For this review, take the finished solid that the model builds, in its own axes (mm). A direction names the side the tool comes from. Round coordinates to 2 decimals unless told otherwise and drop trailing zeros. Loops run counter-clockwise (first coordinate to the right, second up) from the corner with the lowest first, then second, coordinate; pieces in that order, holes last.
1) Mouldability with a two-part tool opening along X and no side actions: class faces 1 (the cylindrical face through (-26, 84, 46)), 2 (the cylindrical face through (4.99, 81.15, 45.94)), 3 (the flat face through (0, 44, 50)) as pulls with the +X half, pulls with the -X half, needs draft (parallel to the pull), parting line crosses it, or undercut.
2) Take a section at B-B (x = -3). State the section outline as (y, z) points.
3) Wall thickness on L1, parallel to Y at x = 5.5, z = 19.5; L2, parallel to Z at x = -15.5, y = 79.5; L3, parallel to X at y = 14.5, z = 48: over which ranges is each line inside the solid? List them lowest first.
4) Take a section at D-D (y = 24.5). State the section outline as (x, z) points.
5) Take a section at C-C (z = 15). State the section outline as (x, y) points, then the cut area to 3 significant figures.
6) Insertion check: pin 1 (5 mm diameter, centred on x = -10, y = 15, fed in from +Z); pin 2 (9 mm diameter, centred on x = -24.5, y = 73.5, fed in from +Z); pin 3 (2.5 mm diameter, centred on x = 0.5, y = -2.5, fed in from -Z); pin 4 (5.5 mm diameter, centred on y = -2, z = 14, fed in from -X). Each pin has a flat end and moves straight along its axis. Give the tip position at first contact, or say it passes through.
7) Take a section at A-A (y = 72.5). State the section outline as (x, z) points, then the cut area to 3 significant figures.
8) Tool access review of faces 4 (the flat face through (-48, 72, 46)), 5 (the flat face through (-37, 72, 49.025)), 6 (the cylindrical face through (-26, 60, 46)), 7 (the flat face through (-37, 72, 43.025)): name each direction out of +Z, -Z, +X, -X, +Y, -Y from which nothing blocks a thin tool from reaching the whole face with its end or side.
```python
from build123d import *

# Parameters (mm, degrees)
ARM_FEATURE_SKETCH_W = 16
ARM_FEATURE_SKETCH_H = 8
ARM_FEATURE_DEPTH    = 50
TAB_FEATURE_SKETCH_W = 8
TAB_FEATURE_SKETCH_H = 25
TAB_FEATURE_DEPTH    = 5
LEG_FEATURE_SKETCH_W = 16
LEG_FEATURE_SKETCH_H = 8
LEG_FEATURE_DEPTH    = 80
SLOT_FEATURE_DEPTH   = 42
STRAP_FEATURE_DEPTH  = 6
STRAP_CUT_SKETCH_W   = 4
STRAP_CUT_SKETCH_H   = 20
STRAP_CUT_DEPTH      = 6
FILLET1_R            = 10
FILLET2_R            = 10
FILLET3_R            = 10


with BuildPart() as part:
    # Arm Feature Sketch → Arm Feature (new body)
    with BuildSketch(Plane.XY):
        Rectangle(ARM_FEATURE_SKETCH_W, ARM_FEATURE_SKETCH_H)
    extrude(amount=ARM_FEATURE_DEPTH)

    # Tab Feature Sketch → Tab Feature (cut)
    with BuildSketch(Plane(origin=(0, -4, 0), x_dir=(1, 0, 0), z_dir=(0, 1, 0))):
        with Locations((0, -12.5)):
            Rectangle(TAB_FEATURE_SKETCH_W, TAB_FEATURE_SKETCH_H)
    extrude(amount=TAB_FEATURE_DEPTH, mode=Mode.SUBTRACT)

    # Leg Feature Sketch → Leg Feature (add)
    with BuildSketch(Plane(origin=(0, 4, 0), x_dir=(1, 0, 0), z_dir=(0, 1, 0))):
        with Locations((0, -46)):
            Rectangle(LEG_FEATURE_SKETCH_W, LEG_FEATURE_SKETCH_H)
    extrude(amount=LEG_FEATURE_DEPTH)

    # Slot Feature Sketch → Slot Feature (add)
    with BuildSketch(Plane(origin=(-8, 0, 0), x_dir=(0, 0, -1), z_dir=(1, 0, 0))):
        with BuildLine():
            Line((-43.025235216, 81), (-43.025235216, 63))
            ThreePointArc((-43.025235216, 63), (-46.025235216, 60), (-49.025235216, 63))
            Line((-49.025235216, 63), (-49.025235216, 81))
            ThreePointArc((-49.025235216, 81), (-46.025235216, 84), (-43.025235216, 81))
        make_face()
    extrude(amount=-SLOT_FEATURE_DEPTH)

    # Strap Feature Sketch → Strap Feature (add)
    with BuildSketch(Plane(origin=(0, 0, 43.025235216), x_dir=(-1, 0, 0), z_dir=(0, 0, -1))):
        with BuildLine():
            Line((44, 63), (44, 81))
            ThreePointArc((44, 81), (50, 87), (56, 81))
            Line((56, 81), (56, 63))
            ThreePointArc((56, 63), (50, 57), (44, 63))
        make_face()
    extrude(amount=-STRAP_FEATURE_DEPTH)

    # Strap Cut Sketch → Strap Cut (cut)
    with BuildSketch(Plane.XY.offset(43.025235216)):
        with Locations((-50, 72)):
            Rectangle(STRAP_CUT_SKETCH_W, STRAP_CUT_SKETCH_H)
    extrude(amount=STRAP_CUT_DEPTH, mode=Mode.SUBTRACT)

    # Fillet1
    fillet1_edges = [part.edges().sort_by_distance(p)[0] for p in [
        (0, -4, 50),
    ]]
    fillet(fillet1_edges, radius=FILLET1_R)

    # Fillet2
    fillet2_edges = [part.edges().sort_by_distance(p)[0] for p in [
        (0, 4, 42),
    ]]
    fillet(fillet2_edges, radius=FILLET2_R)

    # Fillet3
    fillet3_edges = [part.edges().sort_by_distance(p)[0] for p in [
        (8, 84, 46),
    ]]
    fillet(fillet3_edges, radius=FILLET3_R)


solid = part.part
```
Response:
1. face 1: undercut
1. face 2: pulls with the +X half
1. face 3: needs draft
2. outline: (-4, 25) - (1, 25) - (1, 0) - (4, 0) - (4, 32) arc R10 cw to (14, 42) - (84, 42) - (84, 50) - (6, 50) arc R10 ccw to (-4, 40) - close
3. L1: y = -4 to 4
3. L2: z = 43.03 to 49.03
3. L3: x = -8 to 8
4. outline: (-8, 42) - (8, 42) - (8, 50) - (-8, 50) - close
5. outline: (-8, -4) - (-4, -4) - (-4, 1) - (4, 1) - (4, -4) - (8, -4) - (8, 4) - (-8, 4) - close
5. area: 88.0 mm2
6. pin 1: stops at z = 50
6. pin 2: stops at z = 49.03
6. pin 3: stops at z = 25
6. pin 4: stops at x = -8
7. outline: (-56, 43.03) - (-52, 43.03) - (-52, 49.03) - (-56, 49.03) - close; (-48, 43.03) - (-8, 43.03) - (-8, 42) - (8, 42) - (8, 50) - (-8, 50) - (-8, 49.03) - (-48, 49.03) - close
7. area: 392 mm2
8. face 4: +Z, -Z
8. face 5: +Z, -X, +Y, -Y
8. face 6: -Y
8. face 7: -Z, -X, +Y, -Y
